from build123d import *

# Parameters (mm, degrees)
F0_R     = 12.5
F1_DEPTH = 5
F2_R     = 4.99999
F3_T     = 2.5
F4_R     = 1.5
F5_DEPTH = 25
F6_W     = 2
F6_H     = 2
F7_DEPTH = 5
F8_W     = 2
F8_H     = 2
F9_DEPTH = 10


# Not quite as in the source:
# - a fillet or chamfer is up to 0.001 mm smaller than in the source, because OpenCascade refuses the exact size
# - a shell that OpenCascade refuses in one call is made with other operations: the cavity is built on its own and cut out


with BuildPart() as f1:
    # F0 (on Top) → F1 (new body)
    with BuildSketch(Plane.XY):
        Circle(F0_R)
    extrude(amount=F1_DEPTH)

    # F2 (radius 5 in the source; OpenCascade refuses exactly that, so slightly less here)
    f2_edges = [f1.edges().sort_by_distance(p)[0] for p in [
        (-12.5, 0, 5),
    ]]
    fillet(f2_edges, radius=F2_R)

    # F3: shell of thickness 2.5, made by hand


with BuildPart() as f3_core1:
    # F3_t2: copy of F1
    add(f1.part)

    # the walls: a layer under each face that stays
    f3_faces = [f3_core1.faces().sort_by_distance(p)[0] for p in [
        (-12.5, 0, 5e-06),
        (-11.0355368349, 0, 3.5355368349),
        (0, 0, 5),
    ]]
    thicken(f3_faces, amount=-F3_T, mode=Mode.SUBTRACT)


with BuildPart() as f1_1:
    add(f1.part)

    # what is left inside the walls is the cavity
    f3_cavity = [f3_core1.part.solids().sort_by_distance(p)[0] for p in [
        (0, -3.333333, 0.025),
    ]]
    add(f3_cavity, mode=Mode.SUBTRACT)

    # F4 (on face) → F5 (cut)
    with BuildSketch(Plane.XY.offset(5)):
        Circle(F4_R)
    extrude(amount=-F5_DEPTH, mode=Mode.SUBTRACT)

    # F6 (on face) → F7 (join)
    with BuildSketch(Plane.XY.offset(5)):
        with Locations((4, 0)):
            Rectangle(F6_W, F6_H)
        with Locations((-4, 0)):
            Rectangle(F6_W, F6_H)
    extrude(amount=F7_DEPTH)

    # F8 (on face) → F9 (join)
    with BuildSketch(Plane.YZ.offset(5)):
        with Locations((0, 9)):
            Rectangle(F8_W, F8_H)
    extrude(amount=-F9_DEPTH)


solid = f1_1.part
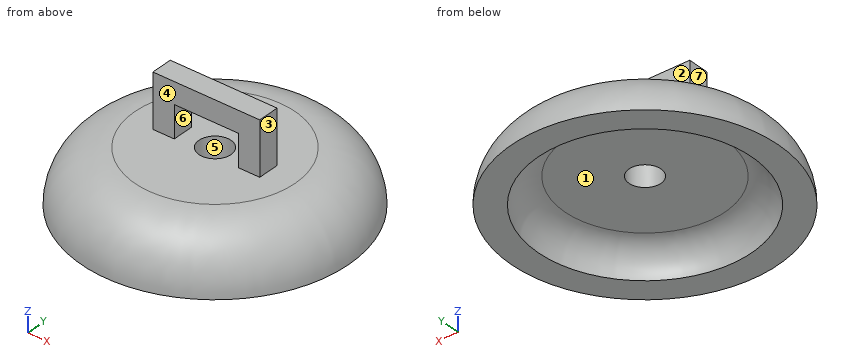
The listing builds one solid part. Answer for the finished solid, in the listing's coordinates (mm). Face numbers are marked on the shaded views. A direction names the side the tool comes from. Coordinates: 2 decimals unless noted, no trailing zeros. Write each loop counter-clockwise with the first axis right and the second up, starting at its lowest first coordinate (ties: lowest second). Pieces come first, ordered by that corner, then holes. Notation, with made-up numbers: M 30,-35 L 72,-35 A13 ccw 72,-17 Z; hole C 73,-23 d5. An arc over 180 degrees is marked long. Use one line per item in the form item = value.
Item 1: For the marked faces 4, 5, 6 and 7, determine the directions among +Z, -Z, +X, -X, +Y, -Y from which every point of the face is accessible in a straight line to the end or side of a thin tool.
Model answer:
face_4 = +Z, +X, -X, -Y
face_5 = -Z
face_6 = +Y, -Y
face_7 = +Z, -X, +Y, -Y
Item 2: Find section D-D, the plane z = 4. Give the vertices of the cut face in (x, y).
Model answer:
outline = C 0,0 d21; hole C 0,0 d3
Item 3: Find section B-B, the plane z = 7.5. Give the vertices of the cut face in (x, y), plus the area to 3 significant figures.
Model answer:
outline = M -5,-1 L -3,-1 L -3,1 L -5,1 Z; M 3,-1 L 5,-1 L 5,1 L 3,1 Z
area = 8.00 mm2
Item 4: Given P1, Ø4, axis at x = -1.5, z = 8.5, coming from the +Y side; P2, Ø1.5, axis at y = 6.5, z = 2.5, coming from the +X side; P3, Ø1.6, axis at y = 0, z = 6.5, coming from the -X side, each flat-ended and moving along its own axis, determine where each tip first touches the part or whether it passes through.
Model answer:
P1 = 1
P2 = 10.52
P3 = -5
Item 5: Find section A-A, the plane x = 0. Give the number of separate pieces and of enclosed holes in the cut face, plus the area to 3 significant figures.
Model answer:
separate_pieces = 3
enclosed_holes = 0
area = 63.5 mm2
Item 6: The mould has two halves that part along Y. Classify the marked faces 1, 2 and 3: released by +Y, released by -Y, zero draft, split by the parting line, or undercut.
Model answer:
face_1 = undercut
face_2 = released by +Y
face_3 = zero draft
Item 7: Find the intervals of material crossed by probe 1 along Z at (x, y) = (2.25, -6.5); probe 2 along X at (y, z) = (5, 1.75); probe 3 along Z at (x, y) = (2.75, 11.5), in increasing order.
Model answer:
probe_1 = 2.5 to 5
probe_2 = -11.11 to -7.82, 7.82 to 11.11
probe_3 = 0 to 2.51
